from build123d import *

# Parameters (mm, degrees)
F0_W     = 63.246
F0_H     = 63.246
F1_DEPTH = 63.5
F2_SIZE  = 9.525
F3_W     = 73.66
F3_H     = 73.66
F4_DEPTH = 9.525
F5_SIZE  = 12.7
F6_R     = 2.54
F7_SIZE  = 1.27
F8_R     = 9.525
F9_DEPTH = 68.454
F11_D    = 12.7
F13_D    = 7.9375


# Not quite as in the source:
# - a length typed as a fraction of an inch, garbled in the dataset ("3 / 203.2 mm" for 3/8 in), is restored


with BuildPart() as f1:
    # F0 (on Top) → F1 (new body)
    with BuildSketch(Plane.XY):
        Rectangle(F0_W, F0_H)
    extrude(amount=-F1_DEPTH)

    # F2
    f2_edges = [f1.edges().sort_by_distance(p)[0] for p in [
        (-31.623, -31.623, -31.75),
        (-31.623, 31.623, -31.75),
        (31.623, -31.623, -31.75),
        (31.623, 31.623, -31.75),
    ]]
    chamfer(f2_edges, length=F2_SIZE)

    # F3 (on face) → F4 (join)
    with BuildSketch(Plane.XY):
        Rectangle(F3_W, F3_H)
    extrude(amount=F4_DEPTH)

    # F5
    f5_edges = [f1.edges().sort_by_distance(p)[0] for p in [
        (36.83, -36.83, 4.7625),
        (-36.83, -36.83, 4.7625),
        (36.83, 36.83, 4.7625),
        (-36.83, 36.83, 4.7625),
    ]]
    chamfer(f5_edges, length=F5_SIZE)

    # F6
    f6_edges = [f1.edges().sort_by_distance(p)[0] for p in [
        (-24.13, -36.83, 4.7625),
        (24.13, -36.83, 4.7625),
        (36.83, -24.13, 4.7625),
        (-36.83, -24.13, 4.7625),
        (36.83, 24.13, 4.7625),
        (24.13, 36.83, 4.7625),
        (-24.13, 36.83, 4.7625),
        (-36.83, 24.13, 4.7625),
        (-22.098, 31.623, -31.75),
        (-31.623, 22.098, -31.75),
        (22.098, 31.623, -31.75),
        (31.623, 22.098, -31.75),
        (-31.623, -22.098, -31.75),
        (-22.098, -31.623, -31.75),
        (31.623, -22.098, -31.75),
        (22.098, -31.623, -31.75),
    ]]
    fillet(f6_edges, radius=F6_R)

    # F7
    f7_edges = [f1.edges().sort_by_distance(p)[0] for p in [
        (-30.48, 30.48, 9.525),
        (-31.623, 0, -63.5),
    ]]
    chamfer(f7_edges, length=F7_SIZE)

    # F8 (on face) → F9 (cut, through all)
    with BuildSketch(Plane(origin=(-31.623, 0, 0), x_dir=(0, -1, 0), z_dir=(-1, 0, 0))):
        with Locations((0, -51.435)):
            Circle(F8_R)
    extrude(amount=-F9_DEPTH, mode=Mode.SUBTRACT)

    # F11 (through all)
    with Locations(Plane.XY.offset(9.525)):
        with Locations((0, 0)):
            Hole(F11_D / 2)

    # F13 (through all)
    with Locations(Plane.YZ.offset(31.623)):
        with Locations((0, -19.05)):
            Hole(F13_D / 2)


solid = f1.part
For this review, take the finished solid that the model builds, in its own axes (mm). A direction names the side the tool comes from. Give positions to 0.01 mm unless a question says otherwise; leave off trailing zeros. Order: outer loops, then holes, each group sorted by start corner. A loop starts at its lowest first (then second) coordinate and runs counter-clockwise, first axis right, second up. Notation, with made-up numbers: (39.25, 79.25) - (60.25, 79.25) arc R13 cw to (60.25, 104.25) - close; hole circle Ø4 at (-5, 33). An arc over 180 degrees is marked (long way). Answer as a JSON object with one key per item and string values. Group by question number.
Item 1: Draft analysis for pull direction X (two halves, no side actions). For faces 1 (the flat face through (26.8, 26.92, -30.68)), 2 (the flat face through (-26.461, 26.349, -62.874)), 3 (the flat face through (0, 8, 9.525)), state which applies: pulls with the +X half, pulls with the -X half, needs draft (parallel to the pull), parting line crosses it, or undercut.
Item 2: Machinability: for faces 4 (the flat face through (30.56, 30.4, 4.07)), 5 (the flat face through (-31.623, 0, -31)), 6 (the flat face through (0, 33, 0)), 7 (the flat face through (26.92, -26.8, -30.68)), 8 (the flat face through (-26.8, 26.92, -30.68)), which of the approach directions +Z, -Z, +X, -X, +Y, -Y give a long, thin tool a straight path to every point of the face, cutting with its end or side? Answer none if there is none.
Item 3: Take a section at C-C on y = 0. Give the number of separate pieces and of enclosed holes in the cut face, and give its area (3 significant figures).
Item 4: Take a section at B-B on z = -19.05. Give the boundary of the cut face in (x, y), and give its area (3 significant figures).
Item 5: Take a section at A-A on x = 0. Give the boundary of the cut face in (y, z) (3 decimals), and give its area (3 significant figures).
Item 6: Take a section at D-D on y = 16. Give the boundary of the cut face in (x, z) (3 decimals).
Item 7: Clearance check with flat-ended pins moving along their axes: pin 1 Ø10.5 at (y, z) = (0, -19.05) entering from +X; pin 2 Ø12.5 at (x, z) = (-1, -24.5) entering from +Y; pin 3 Ø5 at (x, z) = (24, -42.5) entering from -Y. State where each tip first meets the part, or that it passes through.
Item 8: Wall thickness on line 1 along Z through (x, y) = (10.5, 0) (3 decimals); line 2 along Y through (x, z) = (0, -19); line 3 along X through (y, z) = (16, -16): over which ranges is each line inside the solid? List them lowest first.
Reported:
{
 "1": {"face 1": "pulls with the +X half", "face 2": "pulls with the -X half", "face 3": "needs draft"},
 "2": {"face 4": "+Z, -Z, +X, +Y", "face 5": "-Z, -X, +Y, -Y", "face 6": "-Z", "face 7": "-Z, +X, -Y", "face 8": "-Z, -X, +Y"},
 "3": {"separate pieces": "6", "enclosed holes": "0", "area": "2,420 mm^2"},
 "4": {"outline": "(-31.62, -21.05) arc R2.54 ccw to (-30.88, -22.84) - (-22.84, -30.88) arc R2.54 ccw to (-21.05, -31.62) - (21.05, -31.62) arc R2.54 ccw to (22.84, -30.88) - (30.88, -22.84) arc R2.54 ccw to (31.62, -21.05) - (31.62, -3.97) - (4.96, -3.97) arc R6.35 cw to (-4.96, -3.97) - (-31.62, -3.97) - close; (-31.62, 3.97) - (-4.96, 3.97) arc R6.35 cw to (4.96, 3.97) - (31.62, 3.97) - (31.62, 21.05) arc R2.54 ccw to (30.88, 22.84) - (22.84, 30.88) arc R2.54 ccw to (21.05, 31.62) - (-21.05, 31.62) arc R2.54 ccw to (-22.84, 30.88) - (-30.88, 22.84) arc R2.54 ccw to (-31.62, 21.05) - close", "area": "3,280 mm^2"},
 "5": {"outline": "(-36.83, 0) - (-31.623, 0) - (-31.623, -62.23) - (-30.353, -63.5) - (-6.35, -63.5) - (-6.35, -58.535) arc R9.525 cw to (-6.35, -44.335) - (-6.35, 9.525) - (-35.56, 9.525) - (-36.83, 8.255) - close; (6.35, -63.5) - (30.353, -63.5) - (31.623, -62.23) - (31.623, 0) - (36.83, 0) - (36.83, 8.255) - (35.56, 9.525) - (6.35, 9.525) - (6.35, -44.335) arc R9.525 cw to (6.35, -58.535) - close", "area": "3,720 mm^2"},
 "6": {"outline": "(-36.83, 0) - (-31.623, 0) - (-31.623, -62.23) - (-30.353, -63.5) - (30.353, -63.5) - (31.623, -62.23) - (31.623, 0) - (36.83, 0) - (36.83, 8.255) - (35.56, 9.525) - (-35.56, 9.525) - (-36.83, 8.255) - close"},
 "7": {"pin 1": "x = 31.62", "pin 2": "y = 31.62", "pin 3": "y = -31.58"},
 "8": {"line 1": "-63.5 to -60.96, -41.91 to -23.019, -15.081 to 9.525", "line 2": "-31.62 to -6.35, 6.35 to 31.62", "line 3": "-31.62 to 31.62"}
}
